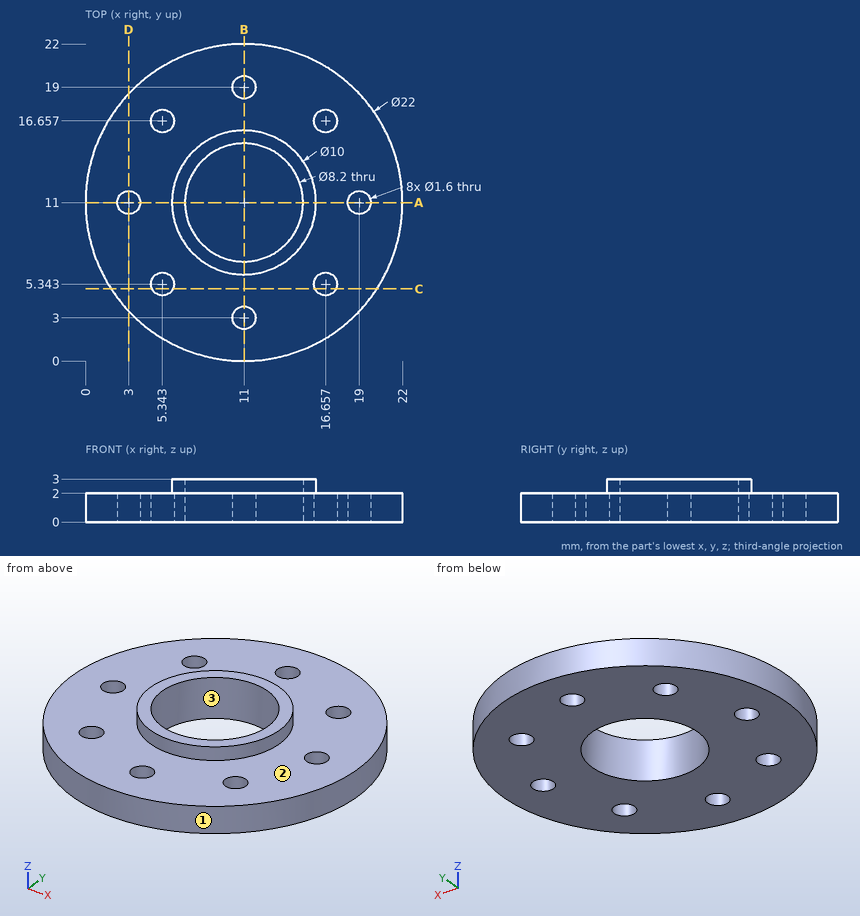
Input: dimensioned drawing with shaded views. Units: mm. Origin: part minimum x, y, z. Round coordinates to 2 decimals unless told otherwise and drop trailing zeros. Write each loop counter-clockwise with the first axis right and the second up, starting at its lowest first coordinate (ties: lowest second). Pieces come first, ordered by that corner, then holes. Notation, with made-up numbers: (-16.75, 23) -> (10.25, 23) arc R20 ccw to (10.25, 53) -> close; hole circle Ø10 at (39.5, -3.75). An arc over 180 degrees is marked (long way). Use CSV: the item, a comma, the result in double quotes. Start each with the question number.
Q1. Section C-C (y = 5). Return loops of the section in (x, z), plus the area to 3 significant figures.
Q2. Line query: L1, parallel to X at y = 10.5, z = 1.45 (1 decimal); L2, parallel to Y at x = 16.25, z = 1.2; L3, parallel to Y at x = 17, z = 1. Output: solid intervals per line, ascending.
Q3. Section A-A (y = 11). Return loops of the section in (x, z), plus the area to 3 significant figures.
Q4. First-contact query: pin 1 Ø1.4 at (x, y) = (19, 11) entering from -Z; pin 2 Ø1 at (x, z) = (4, 0.5) entering from +Y; pin 3 Ø1.5 at (x, z) = (13, 2) entering from -Y; pin 4 Ø2 at (x, y) = (11, 19) entering from +Z. Flat tips, straight axial feed; report the tip coordinate or a pass-through.
Q5. Pull-direction query (Y, two-part tool) for the marked faces 1, 2 and 3; classes: pulls with the +Y half, pulls with the -Y half, needs draft (parallel to the pull), parting line crosses it, or undercut.
Q6. Section D-D (x = 3). Return loops of the section in (y, z), plus the area to 3 significant figures.
Result sheet:
1,outline,"(1.78, 0) -> (4.62, 0) -> (4.62, 2) -> (1.78, 2) -> close; (6.07, 0) -> (15.93, 0) -> (15.93, 2) -> (6.07, 2) -> close; (17.38, 0) -> (20.22, 0) -> (20.22, 2) -> (17.38, 2) -> close"
1,area,"31.1 mm²"
2,L1,"0 to 2.4, 3.6 to 6.9, 15.1 to 18.4, 19.6 to 22"
2,L2,"1.33 to 4.65, 6.03 to 15.97, 17.35 to 20.67"
2,L3,"1.78 to 4.62, 6.07 to 15.93, 17.38 to 20.22"
3,outline,"(0, 0) -> (2.2, 0) -> (2.2, 2) -> (0, 2) -> close; (3.8, 0) -> (6.9, 0) -> (6.9, 3) -> (6, 3) -> (6, 2) -> (3.8, 2) -> close; (15.1, 0) -> (18.2, 0) -> (18.2, 2) -> (16, 2) -> (16, 3) -> (15.1, 3) -> close; (19.8, 0) -> (22, 0) -> (22, 2) -> (19.8, 2) -> close"
3,area,"23.0 mm²"
4,pin 1,"through"
4,pin 2,"y = 19.87"
4,pin 3,"y = 0.07"
4,pin 4,"z = 2"
5,face 1,"parting line crosses it"
5,face 2,"needs draft"
5,face 3,"undercut"
6,outline,"(3.45, 0) -> (10.2, 0) -> (10.2, 2) -> (3.45, 2) -> close; (11.8, 0) -> (18.55, 0) -> (18.55, 2) -> (11.8, 2) -> close"
6,area,"27.0 mm²"
